Read the model definition and answer for the solid it produces. Units are mm, in the model's axes. A direction names the side the tool comes from. Coordinates: 2 decimals unless noted, no trailing zeros. Order: outer loops, then holes, each group sorted by start corner. A loop starts at its lowest first (then second) coordinate and runs counter-clockwise, first axis right, second up. Notation, with made-up numbers: M 58.5,56 L 101.5,56 A32 ccw 101.5,88 Z; hole C -25,79 d11. An arc over 180 degrees is marked long. Write each question's results on one line, items separated by ' | '.
```python
from build123d import *

# Parameters (mm, degrees)
SKETCH1_R           = 21
SKETCH1_W           = 5
SKETCH1_H           = 5
BOSS_EXTRUDE1_DEPTH = 2
SKETCH2_W           = 3.8
SKETCH2_H           = 3.8
BOSS_EXTRUDE2_DEPTH = 5
CUT_EXTRUDE1_REACH  = 49.263
SKETCH3_R           = 1.5
CUT_EXTRUDE2_REACH  = 49.009
FILLET1_R           = 0.7


with BuildPart() as part:
    # Sketch1 → Boss-Extrude1 (new body)
    # profile 1 of 6: a face of its own
    with BuildSketch(Plane(origin=(0, 0, 0), x_dir=(1, 0, 0), z_dir=(0, 1, 0))):
        Circle(SKETCH1_R)
    # profile 2 of 6: a face of its own
    with BuildSketch(Plane(origin=(0, 0, 0), x_dir=(1, 0, 0), z_dir=(0, 1, 0))):
        with BuildLine():
            Line((0, 0), (-17.886625066, -21.898189918))
            ThreePointArc((-17.886625066, -21.898189918), (-17.5, -30.310889132), (-10.021076233, -26.439366654))
            Line((-10.021076233, -26.439366654), (0, 0))
        make_face()
        with Locations((-15, -25.980762114)):
            Rectangle(SKETCH1_W, SKETCH1_H, mode=Mode.SUBTRACT)
    # profile 3 of 6: a face of its own
    with BuildSketch(Plane(origin=(0, 0, 0), x_dir=(1, 0, 0), z_dir=(0, 1, 0))):
        Circle(SKETCH1_R)
    # profile 4 of 6: a face of its own
    with BuildSketch(Plane(origin=(0, 0, 0), x_dir=(1, 0, 0), z_dir=(0, 1, 0))):
        with BuildLine():
            Line((0, 0), (27.907701299, -4.541176736))
            ThreePointArc((27.907701299, -4.541176736), (35, 0), (27.907701299, 4.541176736))
            Line((27.907701299, 4.541176736), (0, 0))
        make_face()
        Polygon((29.084936491, -3.415063509), (26.584936491, 0.915063509), (30.915063509, 3.415063509), (33.415063509, -0.915063509), align=None, mode=Mode.SUBTRACT)
    # profile 5 of 6: a face of its own
    with BuildSketch(Plane(origin=(0, 0, 0), x_dir=(1, 0, 0), z_dir=(0, 1, 0))):
        Circle(SKETCH1_R)
    # profile 6 of 6: a face of its own
    with BuildSketch(Plane(origin=(0, 0, 0), x_dir=(1, 0, 0), z_dir=(0, 1, 0))):
        with BuildLine():
            Line((0, 0), (-10.021076233, 26.439366654))
            ThreePointArc((-10.021076233, 26.439366654), (-17.5, 30.310889132), (-17.886625066, 21.898189918))
            Line((-17.886625066, 21.898189918), (0, 0))
        make_face()
        Polygon((-11.584936491, 26.895825623), (-14.084936491, 22.565698604), (-18.415063509, 25.065698604), (-15.915063509, 29.395825623), align=None, mode=Mode.SUBTRACT)
    extrude(amount=BOSS_EXTRUDE1_DEPTH)

    # Sketch2 → Boss-Extrude2 (add)
    with BuildSketch(Plane(origin=(0, 2, 0), x_dir=(1, 0, 0), z_dir=(0, 1, 0))):
        Rectangle(SKETCH2_W, SKETCH2_H)
    extrude(amount=BOSS_EXTRUDE2_DEPTH)

    # Sketch3 → Cut-Extrude1 (cut, up to next)
    with BuildSketch(Plane(origin=(0, 7, 0), x_dir=(1, 0, 0), z_dir=(0, 1, 0)), mode=Mode.PRIVATE) as cut_extrude1_sk1:
        with Locations(Location((0, 0, 0), (0, 0, 270))):
            Circle(SKETCH3_R)
    cut_extrude1_tool1 = extrude(cut_extrude1_sk1.sketch, amount=-CUT_EXTRUDE1_REACH, mode=Mode.PRIVATE) & part.part
    add(cut_extrude1_tool1.solids().sort_by_distance((0, 7, 0))[0], mode=Mode.SUBTRACT)

    # Sketch4 → Cut-Extrude2 (cut, up to next)
    with BuildSketch(Plane(origin=(0, 2, 0), x_dir=(1, 0, 0), z_dir=(0, 1, 0)), mode=Mode.PRIVATE) as cut_extrude2_sk1:
        with BuildLine():
            Line((-3.620274752, -0.735), (-17.599715907, -9.5))
            ThreePointArc((-17.599715907, -9.5), (-20, 0), (-17.599715907, 9.5))
            Line((-17.599715907, 9.5), (-3.620274752, 0.735))
            ThreePointArc((-3.620274752, 0.735), (-3.694132412, 0), (-3.620274752, -0.735))
        make_face()
    cut_extrude2_tool1 = extrude(cut_extrude2_sk1.sketch, amount=-CUT_EXTRUDE2_REACH, mode=Mode.PRIVATE) & part.part
    add(cut_extrude2_tool1.solids().sort_by_distance((-13.664779, 2, 0))[0], mode=Mode.SUBTRACT)

    # Fillet1
    # the kernel refuses this fillet: 0.7 mm, written as the material it takes off along each edge
    with BuildSketch(Plane(origin=(-1.9, 7, 3.65), x_dir=(0, -1, 0), z_dir=(0, 0, -1)), Plane(origin=(3.65, 7, 1.9), x_dir=(0, -1, 0), z_dir=(-1, 0, 0)), Plane(origin=(1.9, 7, -3.65), x_dir=(0, -1, 0), z_dir=(0, 0, 1)), Plane(origin=(-3.65, 7, -1.9), x_dir=(0, -1, 0), z_dir=(1, 0, 0))) as fillet1_piece_1:
        with BuildLine():
            CenterArc((FILLET1_R, -FILLET1_R), FILLET1_R, 90, 90)
            Line((0, -FILLET1_R), (0, 0))
            Line((0, 0), (FILLET1_R, 0))
        make_face()
    extrude(amount=7.3, mode=Mode.SUBTRACT)


solid = part.part
```
(1) For faces 1 (the flat face through (1.9, 4, 0)), 2 (the flat face through (27.85, 0.99, 1.28)), 3 (the flat face through (24.368, 0.986, -3.965)), 4 (the flat face through (-1.9, 4, 0)), determine the directions among +Z, -Z, +X, -X, +Y, -Y from which every point of the face is accessible in a straight line to the end or side of a thin tool.
Conclusion:
face 1: +Z, -Z, +X, +Y | face 2: +Y, -Y | face 3: -Z, +Y, -Y | face 4: +Z, -Z, -X, +Y
(2) Straight lines are drawn through the part: line 1 (X direction, y = 4, z = 0); line 2 (Y direction, x = 10, z = -2). For each, find the intervals that lie inside material, in ascending order.
Conclusion:
line 1: -1.9 to -1.5, 1.5 to 1.9 | line 2: 0 to 2
(3) The part is cut by section D-D, the plane z = -6.5. Write down the section's boundary in (x, y).
Conclusion:
outline: M -19.97,0 L -18.91,0 L -18.91,2 L -19.97,2 Z; M -12.81,0 L 19.97,0 L 19.97,2 L -12.81,2 Z
(4) The mould has two halves that part along X. Classify faces 5 (the flat face through (-15.6, 1, -19.1)), 6 (the flat face through (-12.82, 0.99, -24.76)), 7 (the flat face through (7, 0, 0)), 8 (the flat face through (-8.714, 0.986, -22.99)): pulls with the +X half, pulls with the -X half, needs draft (parallel to the pull), parting line crosses it, or undercut.
Conclusion:
face 5: pulls with the -X half | face 6: undercut | face 7: needs draft | face 8: undercut
(5) The part is cut by section C-C, the plane y = 1. Count the separate pieces of the cut face and the enclosed holes in it, then the cut area to 3 significant figures.
Conclusion:
separate pieces: 1 | enclosed holes: 5 | area: 1,480 mm²
(6) The part is cut by section A-A, the plane z = 0. Write down the section's boundary in (x, y), then the cut area to 3 significant figures.
Conclusion:
outline: M -21,0 L -20,0 L -20,2 L -21,2 Z; M -3.69,0 L -1.5,0 L -1.5,6.93 A0.7 ccw -1.9,6.3 L -1.9,2 L -3.69,2 Z; M 1.5,0 L 27.11,0 L 27.11,2 L 1.9,2 L 1.9,6.3 A0.7 ccw 1.5,6.93 Z; M 32.89,0 L 35,0 L 35,2 L 32.89,2 Z | area: 65.6 mm²
(7) The part is cut by section B-B, the plane x = 0. Write down the section's boundary in (y, z).
Conclusion:
outline: M 0,-21 L 2,-21 L 2,-1.9 L 6.3,-1.9 A0.7 ccw 6.93,-1.5 L 0,-1.5 Z; M 0,1.5 L 6.93,1.5 A0.7 ccw 6.3,1.9 L 2,1.9 L 2,21 L 0,21 Z
(8) Given pin 1 (2.5 mm diameter, centred on x = 0, z = 0, fed in from +Y); pin 2 (1 mm diameter, centred on x = 11.5, z = 4.5, fed in from -Y); pin 3 (0.6 mm diameter, centred on y = 1.5, z = 26, fed in from -X); pin 4 (4 mm diameter, centred on x = -0.5, y = 3.5, fed in from -Z), each flat-ended and moving along its own axis, determine where each tip first touches the part or whether it passes through.
Conclusion:
pin 1: through | pin 2: y = 0 | pin 3: x = -20 | pin 4: z = -21
